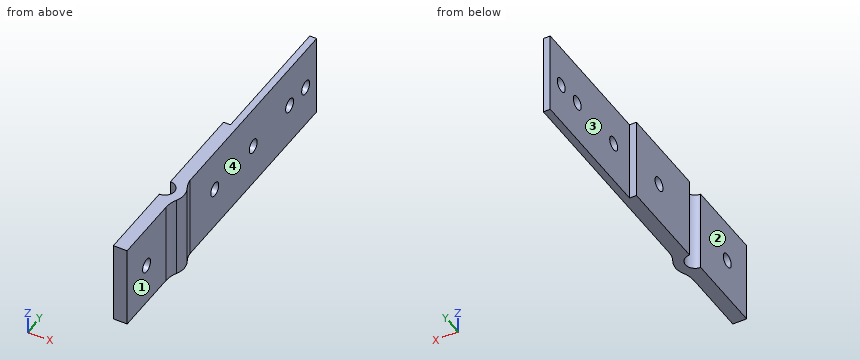
```python
from build123d import *

# Parameters (mm, degrees)
SKETCH1_R           = 7
SKETCH1_R_2         = 2.5
BOSS_EXTRUDE1_DEPTH = 30
SKETCH2_W           = 5
SKETCH2_H           = 80
BOSS_EXTRUDE2_DEPTH = 30
SKETCH3_W           = 4.993372703
SKETCH3_H           = 5.857886356
BOSS_EXTRUDE3_DEPTH = 30
FILLET1_R           = 10
SKETCH4_R           = 2.5
CUT_EXTRUDE1_DEPTH  = 30
SKETCH5_W           = 18.483603476
SKETCH5_H           = 15.568617645
CUT_EXTRUDE2_DEPTH  = 30
SKETCH6_W           = 30
SKETCH6_H           = 30
BOSS_EXTRUDE4_DEPTH = 5
FILLET2_R           = 10
SKETCH7_R           = 2.5
CUT_EXTRUDE3_DEPTH  = 5
SKETCH8_R           = 3.5
CUT_EXTRUDE4_DEPTH  = 45
SKETCH9_W           = 2.5
SKETCH9_H           = 50
CUT_EXTRUDE5_DEPTH  = 50


with BuildPart() as part:
    # Sketch1 → Boss-Extrude1 (new body)
    with BuildSketch(Plane.XY):
        Circle(SKETCH1_R)
        Circle(SKETCH1_R_2, mode=Mode.SUBTRACT)
    extrude(amount=BOSS_EXTRUDE1_DEPTH)



with BuildPart() as body_2:
    # Sketch2 → Boss-Extrude2 (new body)
    with BuildSketch(Plane.XY.offset(30)):
        with Locations((2.5, 47)):
            Rectangle(SKETCH2_W, SKETCH2_H)
    extrude(amount=-BOSS_EXTRUDE2_DEPTH)


with BuildPart() as part_1:
    add(part.part)

    add(body_2.part)  # Boss-Extrude3 merges body 2
    # Sketch3 → Boss-Extrude3 (add)
    with BuildSketch(Plane.XY.offset(30)):
        with Locations((2.496686352, 6.222987156)):
            Rectangle(SKETCH3_W, SKETCH3_H)
    extrude(amount=-BOSS_EXTRUDE3_DEPTH)

    # Fillet1
    # the kernel refuses this fillet: 10 mm, written as the material it adds along each edge
    with BuildSketch(Plane(origin=(4.993372703, 4.905734302, 30), x_dir=(0.5953030074324868, -0.8035012939266724, 0), z_dir=(0, 0, -1))) as fillet1_piece_1:
        with BuildLine():
            CenterArc((3.322951104, -9.903685446), FILLET1_R, 97.958528589, 22.079165002)
            Line((-1.682745198, -1.246722668), (-1.782859124, -1.073583413))
            ThreePointArc((-1.782859124, -1.073583413), (-0.9604332, -0.462661075), (-0.119060601, 0.160700259))
            Line((-0.119060601, 0.160700259), (0.027691259, 0.198073709))
            ThreePointArc((0.027691259, 0.198073709), (0.969194072, 0.132579812), (1.910696885, 0.198073709))
            Line((1.910696885, 0.198073709), (1.938388144, 0))
        make_face()
    extrude(amount=30)

    # Sketch4 → Cut-Extrude1 (cut)
    with BuildSketch(Plane(origin=(5, 0, 0), x_dir=(0, 0, -1), z_dir=(1, 0, 0))):
        with Locations((-15, 22.761745694)):
            Circle(SKETCH4_R)
        with Locations((-15, 47)):
            Circle(SKETCH4_R)
        with Locations((-15, 69.953924783)):
            Circle(SKETCH4_R)
        with Locations((-15, 80.047807532)):
            Circle(SKETCH4_R)
    extrude(amount=-CUT_EXTRUDE1_DEPTH, mode=Mode.SUBTRACT)

    # Sketch5 → Cut-Extrude2 (cut)
    with BuildSketch(Plane(origin=(0, 0, 0), x_dir=(-1, 0, 0), z_dir=(0, 0, -1))):
        with Locations((9.241801738, -0.784308822)):
            Rectangle(SKETCH5_W, SKETCH5_H)
    extrude(amount=-CUT_EXTRUDE2_DEPTH, mode=Mode.SUBTRACT)

    # Sketch6 → Boss-Extrude4 (add)
    with BuildSketch(Plane.ZY):
        with Locations((15, -17.5)):
            Rectangle(SKETCH6_W, SKETCH6_H)
    extrude(amount=-BOSS_EXTRUDE4_DEPTH)

    # Fillet2
    fillet2_edges = [part_1.edges().sort_by_distance(p)[0] for p in [
        (5, -4.898979486, 15),
    ]]
    fillet(fillet2_edges, radius=FILLET2_R)

    # Sketch7 → Cut-Extrude3 (cut)
    with BuildSketch(Plane(origin=(5, 0, 0), x_dir=(0, 0, -1), z_dir=(1, 0, 0))):
        with Locations((-15, -20.25)):
            Circle(SKETCH7_R)
    extrude(amount=-CUT_EXTRUDE3_DEPTH, mode=Mode.SUBTRACT)

    # Sketch8 → Cut-Extrude4 (cut)
    with BuildSketch(Plane(origin=(0, 0, 0), x_dir=(-1, 0, 0), z_dir=(0, 0, -1))):
        Circle(SKETCH8_R)
    extrude(amount=-CUT_EXTRUDE4_DEPTH, mode=Mode.SUBTRACT)

    # Sketch9 → Cut-Extrude5 (cut)
    with BuildSketch(Plane(origin=(0, 0, 0), x_dir=(-1, 0, 0), z_dir=(0, 0, -1))):
        with Locations((-1.25, 62)):
            Rectangle(SKETCH9_W, SKETCH9_H)
    extrude(amount=-CUT_EXTRUDE5_DEPTH, mode=Mode.SUBTRACT)


solid = part_1.part
```
Design review of the part built by this model. Coordinates are the model's own, in mm. Face numbers are marked on the shaded views. A direction names the side the tool comes from. Give positions to 0.01 mm unless a question says otherwise; leave off trailing zeros. Write each loop counter-clockwise with the first axis right and the second up, starting at its lowest first coordinate (ties: lowest second). Pieces come first, ordered by that corner, then holes. Notation, with made-up numbers: (50.25, 84.25) - (71.25, 84.25) arc R29 cw to (71.25, 107.25) - close; hole circle Ø2 at (-8.75, 17). An arc over 180 degrees is marked (long way). Return JSON: item names as keys, results as strings. Group by question number.
(1) To check wall thickness, follow probe 1 along Y at (x, z) = (3.9, 15); probe 2 along Y at (x, z) = (1.1, 15); probe 3 along Y at (x, z) = (2.25, 16). State the ranges of each line that lie inside material, in increasing order.
(2) Insertion check: pin 1 (4 mm diameter, centred on y = 47, z = 15, fed in from -X); pin 2 (6 mm diameter, centred on y = 80.05, z = 15, fed in from +X); pin 3 (15 mm diameter, centred on y = 73.5, z = 16.5, fed in from -X); pin 4 (4 mm diameter, centred on x = 1.5, y = 21.5, fed in from -Z). Each pin has a flat end and moves straight along its axis. Give the tip position at first contact, or say it passes through.
(3) We need section B-B, the plane z = 15. Give the number of separate pieces and of enclosed holes in the cut face, then the cut area to 3 significant figures.
(4) We need section A-A, the plane y = -20.25. Give the boundary of the cut face in (x, z).
(5) We need section D-D, the plane y = 47. Give the boundary of the cut face in (x, z), then the cut area to 3 significant figures.
(6) Machinability: for the marked faces 1, 2, 3 and 4, which of the approach directions +Z, -Z, +X, -X, +Y, -Y give a long, thin tool a straight path to every point of the face, cutting with its end or side? Answer none if there is none.
Reported:
{
 "1": {"probe 1": "y = -32.5 to -22.75, -17.75 to 20.26, 25.26 to 44.5, 49.5 to 67.45, 72.45 to 77.55, 82.55 to 87", "probe 2": "y = -32.5 to -22.75, -17.75 to -3.32, 3.32 to 20.26, 25.26 to 37", "probe 3": "y = -32.5 to -22.54, -17.96 to -2.68, 2.68 to 20.47, 25.05 to 37"},
 "2": {"pin 1": "passes through", "pin 2": "stops at x = 5", "pin 3": "stops at x = 2.5", "pin 4": "stops at z = 0"},
 "3": {"separate pieces": "6", "enclosed holes": "0", "area": "381 mm2"},
 "4": {"outline": "(0, 0) - (5, 0) - (5, 12.5) - (0, 12.5) - close; (0, 17.5) - (5, 17.5) - (5, 30) - (0, 30) - close"},
 "5": {"outline": "(2.5, 0) - (5, 0) - (5, 12.5) - (2.5, 12.5) - close; (2.5, 17.5) - (5, 17.5) - (5, 30) - (2.5, 30) - close", "area": "62.5 mm2"},
 "6": {"face 1": "+Z, -Z, +X, -Y", "face 2": "+Z, -Z, -X, +Y, -Y", "face 3": "+Z, -Z, -X, +Y", "face 4": "+Z, -Z, +X, +Y"}
}
